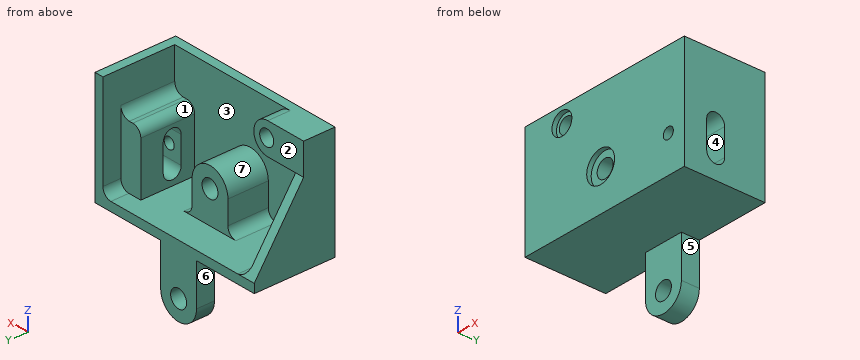
from build123d import *

# Parameters (mm, degrees)
BOSS_EXTRUDE1_DEPTH                                  = 6.35
BOSS_EXTRUDE2_DEPTH                                  = 57.15
BOSS_EXTRUDE3_DEPTH                                  = 44.45
BOSS_EXTRUDE4_DEPTH                                  = 34.925
SKETCH4_R                                            = 14.2875
SKETCH4_R_2                                          = 6.35
BOSS_EXTRUDE5_DEPTH                                  = 12.7
CUT_EXTRUDE1_REACH                                   = 159.28
BOSS_EXTRUDE6_DEPTH                                  = 15.875
CBORE_FOR_M5_CROSS_RECESS_PAN_HEAD_SCREW_D           = 11.2014
CBORE_FOR_M5_CROSS_RECESS_PAN_HEAD_SCREW_CBORE_D     = 15.875
CBORE_FOR_M5_CROSS_RECESS_PAN_HEAD_SCREW_CBORE_DEPTH = 3.175
CBORE_FOR_M5_CROSS_RECESS_PAN_HEAD_S_2_D             = 12.7
CBORE_FOR_M5_CROSS_RECESS_PAN_HEAD_S_2_CBORE_D       = 22.225
CBORE_FOR_M5_CROSS_RECESS_PAN_HEAD_S_2_CBORE_DEPTH   = 3.175
CUT_EXTRUDE3_REACH                                   = 159.28
CUT_EXTRUDE4_REACH                                   = 116.252
SKETCH18_R                                           = 4.0005


with BuildPart() as part:
    # Sketch1 → Boss-Extrude1 (new body)
    with BuildSketch(Plane(origin=(0, 0, 0), x_dir=(1, 0, 0), z_dir=(0, 1, 0))):
        with BuildLine():
            Line((60.325, 16.51822322), (60.325, -28.346886894))
            Line((60.325, -28.346886894), (60.325, -50.8))
            Line((60.325, -50.8), (66.675, -50.8))
            Line((66.675, -50.8), (66.675, 29.21822322))
            Line((66.675, 29.21822322), (-60.325, 29.21822322))
            Line((-60.325, 29.21822322), (-60.325, -50.8))
            Line((-60.325, -50.8), (-53.975, -50.8))
            Line((-53.975, -50.8), (-53.975, -44.45))
            Line((-53.975, -44.45), (-53.975, 16.103113106))
            ThreePointArc((-53.975, 16.103113106), (-51.993545123, 20.886768343), (-47.209889886, 22.86822322))
            Line((-47.209889886, 22.86822322), (-20.6375, 22.86822322))
            Line((-20.6375, 22.86822322), (20.6375, 22.86822322))
            Line((20.6375, 22.86822322), (44.45, 22.86822322))
            Line((44.45, 22.86822322), (53.975, 22.86822322))
            ThreePointArc((53.975, 22.86822322), (58.465128061, 21.00835128), (60.325, 16.51822322))
        make_face()
        with BuildLine():
            Line((60.325, -50.8), (60.325, -28.346886894))
            ThreePointArc((60.325, -28.346886894), (58.343545123, -23.563231657), (53.559889886, -21.58177678))
            Line((53.559889886, -21.58177678), (50.8, -21.58177678))
            ThreePointArc((50.8, -21.58177678), (46.309871939, -19.721904841), (44.45, -15.23177678))
            Line((44.45, -15.23177678), (44.45, 22.86822322))
            Line((44.45, 22.86822322), (20.6375, 22.86822322))
            ThreePointArc((20.6375, 22.86822322), (16.147371939, 21.00835128), (14.2875, 16.51822322))
            Line((14.2875, 16.51822322), (14.2875, 0))
            ThreePointArc((14.2875, 0), (0, -14.2875), (-14.2875, 0))
            Line((-14.2875, 0), (-14.2875, 16.51822322))
            ThreePointArc((-14.2875, 16.51822322), (-16.147371939, 21.00835128), (-20.6375, 22.86822322))
            Line((-20.6375, 22.86822322), (-47.209889886, 22.86822322))
            ThreePointArc((-47.209889886, 22.86822322), (-51.993545123, 20.886768343), (-53.975, 16.103113106))
            Line((-53.975, 16.103113106), (-53.975, -44.45))
            Line((-53.975, -44.45), (-53.975, -50.8))
            Line((-53.975, -50.8), (-47.625, -50.8))
            Line((-47.625, -50.8), (60.325, -50.8))
        make_face()
        with BuildLine():
            Line((-20.6375, 22.86822322), (20.6375, 22.86822322))
            ThreePointArc((20.6375, 22.86822322), (16.147371939, 21.00835128), (14.2875, 16.51822322))
            Line((14.2875, 16.51822322), (14.2875, 0))
            ThreePointArc((14.2875, 0), (0, -14.2875), (-14.2875, 0))
            Line((-14.2875, 0), (-14.2875, 16.51822322))
            ThreePointArc((-14.2875, 16.51822322), (-16.147371939, 21.00835128), (-20.6375, 22.86822322))
        make_face()
        with BuildLine():
            ThreePointArc((53.559889886, -21.58177678), (58.343545123, -23.563231657), (60.325, -28.346886894))
            Line((60.325, -28.346886894), (60.325, 16.51822322))
            ThreePointArc((60.325, 16.51822322), (58.465128061, 21.00835128), (53.975, 22.86822322))
            Line((53.975, 22.86822322), (44.45, 22.86822322))
            Line((44.45, 22.86822322), (44.45, -15.23177678))
            ThreePointArc((44.45, -15.23177678), (46.309871939, -19.721904841), (50.8, -21.58177678))
            Line((50.8, -21.58177678), (53.559889886, -21.58177678))
        make_face()
    extrude(amount=BOSS_EXTRUDE1_DEPTH)

    # Sketch1<4> → Boss-Extrude2 (add)
    with BuildSketch(Plane(origin=(0, 0, 0), x_dir=(1, 0, 0), z_dir=(0, 1, 0))):
        with BuildLine():
            Line((60.325, 16.51822322), (60.325, -28.346886894))
            Line((60.325, -28.346886894), (60.325, -50.8))
            Line((60.325, -50.8), (66.675, -50.8))
            Line((66.675, -50.8), (66.675, 29.21822322))
            Line((66.675, 29.21822322), (-60.325, 29.21822322))
            Line((-60.325, 29.21822322), (-60.325, -50.8))
            Line((-60.325, -50.8), (-53.975, -50.8))
            Line((-53.975, -50.8), (-53.975, -44.45))
            Line((-53.975, -44.45), (-53.975, 16.103113106))
            ThreePointArc((-53.975, 16.103113106), (-51.993545123, 20.886768343), (-47.209889886, 22.86822322))
            Line((-47.209889886, 22.86822322), (-20.6375, 22.86822322))
            Line((-20.6375, 22.86822322), (20.6375, 22.86822322))
            Line((20.6375, 22.86822322), (44.45, 22.86822322))
            Line((44.45, 22.86822322), (53.975, 22.86822322))
            ThreePointArc((53.975, 22.86822322), (58.465128061, 21.00835128), (60.325, 16.51822322))
        make_face()
    extrude(amount=BOSS_EXTRUDE2_DEPTH)

    # Sketch1<5> → Boss-Extrude3 (add)
    with BuildSketch(Plane(origin=(0, 0, 0), x_dir=(1, 0, 0), z_dir=(0, 1, 0))):
        with BuildLine():
            ThreePointArc((53.559889886, -21.58177678), (58.343545123, -23.563231657), (60.325, -28.346886894))
            Line((60.325, -28.346886894), (60.325, 16.51822322))
            ThreePointArc((60.325, 16.51822322), (58.465128061, 21.00835128), (53.975, 22.86822322))
            Line((53.975, 22.86822322), (44.45, 22.86822322))
            Line((44.45, 22.86822322), (44.45, -15.23177678))
            ThreePointArc((44.45, -15.23177678), (46.309871939, -19.721904841), (50.8, -21.58177678))
            Line((50.8, -21.58177678), (53.559889886, -21.58177678))
        make_face()
    extrude(amount=BOSS_EXTRUDE3_DEPTH)

    # Sketch1<6> → Boss-Extrude4 (add)
    with BuildSketch(Plane(origin=(0, 0, 0), x_dir=(1, 0, 0), z_dir=(0, 1, 0))):
        with BuildLine():
            Line((-20.6375, 22.86822322), (20.6375, 22.86822322))
            ThreePointArc((20.6375, 22.86822322), (16.147371939, 21.00835128), (14.2875, 16.51822322))
            Line((14.2875, 16.51822322), (14.2875, 0))
            ThreePointArc((14.2875, 0), (0, -14.2875), (-14.2875, 0))
            Line((-14.2875, 0), (-14.2875, 16.51822322))
            ThreePointArc((-14.2875, 16.51822322), (-16.147371939, 21.00835128), (-20.6375, 22.86822322))
        make_face()
    extrude(amount=BOSS_EXTRUDE4_DEPTH)

    # Sketch4 → Boss-Extrude5 (add)
    # profile 1 of 2: a face of its own
    with BuildSketch(Plane(origin=(0, 57.15, 0), x_dir=(1, 0, 0), z_dir=(0, 1, 0))):
        with BuildLine():
            ThreePointArc((14.2875, 58.801), (0, 44.5135), (-14.2875, 58.801))
            Line((-14.2875, 58.801), (-14.2875, 29.21822322))
            Line((-14.2875, 29.21822322), (14.2875, 29.21822322))
            Line((14.2875, 29.21822322), (14.2875, 58.801))
        make_face()
    # profile 2 of 2: a face of its own
    with BuildSketch(Plane(origin=(0, 57.15, 0), x_dir=(1, 0, 0), z_dir=(0, 1, 0))):
        with Locations((0, 58.801)):
            Circle(SKETCH4_R)
        with Locations(Location((0, 58.801, 0), (0, 0, 270))):
            Circle(SKETCH4_R_2, mode=Mode.SUBTRACT)
    extrude(amount=-BOSS_EXTRUDE5_DEPTH)

    # Sketch5 → Cut-Extrude1 (cut, up to next)
    with BuildSketch(Plane.ZY.offset(60.325), mode=Mode.PRIVATE) as cut_extrude1_sk1:
        Polygon((-22.86822322, 57.15), (28.575, 22.225), (50.8, 22.225), (50.8, 57.15), align=None)
    cut_extrude1_tool1 = extrude(cut_extrude1_sk1.sketch, amount=-CUT_EXTRUDE1_REACH, mode=Mode.PRIVATE) & part.part
    add(cut_extrude1_tool1.solids().sort_by_distance((-60.325, 42.810165, 24.526909))[0], mode=Mode.SUBTRACT)

    # Sketch6 → Boss-Extrude6 (add)
    with BuildSketch(Plane(origin=(0, 6.35, 0), x_dir=(1, 0, 0), z_dir=(0, 1, 0))):
        with BuildLine():
            Line((-31.75, -28.575), (-53.975, -28.575))
            Line((-53.975, -28.575), (-53.975, -50.8))
            Line((-53.975, -50.8), (-31.75, -50.8))
            ThreePointArc((-31.75, -50.8), (-20.6375, -39.6875), (-31.75, -28.575))
        make_face()
    extrude(amount=BOSS_EXTRUDE6_DEPTH)

    # CBORE for M5 Cross Recess Pan Head Screw (through all)
    with Locations(Plane(origin=(0, 0, 0), x_dir=(-1, 0, 0), z_dir=(0, -1, 0))):
        with Locations((30.873227599, -39.973489035)):
            CounterBoreHole(CBORE_FOR_M5_CROSS_RECESS_PAN_HEAD_SCREW_D / 2, CBORE_FOR_M5_CROSS_RECESS_PAN_HEAD_SCREW_CBORE_D / 2, CBORE_FOR_M5_CROSS_RECESS_PAN_HEAD_SCREW_CBORE_DEPTH)

    # CBORE for M5 Cross Recess Pan Head S 2 (through all)
    with Locations(Plane(origin=(0, 0, 0), x_dir=(-1, 0, 0), z_dir=(0, -1, 0))):
        with Locations((0, 0)):
            CounterBoreHole(CBORE_FOR_M5_CROSS_RECESS_PAN_HEAD_S_2_D / 2, CBORE_FOR_M5_CROSS_RECESS_PAN_HEAD_S_2_CBORE_D / 2, CBORE_FOR_M5_CROSS_RECESS_PAN_HEAD_S_2_CBORE_DEPTH)

    # Sketch16 → Cut-Extrude3 (cut, up to next)
    with BuildSketch(Plane(origin=(66.675, 0, 0), x_dir=(0, 0, -1), z_dir=(1, 0, 0)), mode=Mode.PRIVATE) as cut_extrude3_sk1:
        with BuildLine():
            Line((-6.35, 28.575), (12.7, 28.575))
            ThreePointArc((12.7, 28.575), (19.05, 22.225), (12.7, 15.875))
            Line((12.7, 15.875), (-6.35, 15.875))
            ThreePointArc((-6.35, 15.875), (-12.7, 22.225), (-6.35, 28.575))
        make_face()
    cut_extrude3_tool1 = extrude(cut_extrude3_sk1.sketch, amount=-CUT_EXTRUDE3_REACH, mode=Mode.PRIVATE) & part.part
    add(cut_extrude3_tool1.solids().sort_by_distance((66.675, 22.225, -3.175))[0], mode=Mode.SUBTRACT)

    # Sketch18 → Cut-Extrude4 (cut, up to next)
    with BuildSketch(Plane(origin=(0, 0, 0), x_dir=(-1, 0, 0), z_dir=(0, -1, 0)), mode=Mode.PRIVATE) as cut_extrude4_sk1:
        with Locations(Location((-53.975, 3.175, 0), (0, 0, 90))):
            Circle(SKETCH18_R)
    cut_extrude4_tool1 = extrude(cut_extrude4_sk1.sketch, amount=-CUT_EXTRUDE4_REACH, mode=Mode.PRIVATE) & part.part
    add(cut_extrude4_tool1.solids().sort_by_distance((53.975, 0, -3.175))[0], mode=Mode.SUBTRACT)


solid = part.part
Input: part model. Units: mm. Frame: model coordinates. Face numbers are marked on the shaded views. A direction names the side the tool comes from. Round coordinates to 2 decimals unless told otherwise and drop trailing zeros. Order: outer loops, then holes, each group sorted by start corner. A loop starts at its lowest first (then second) coordinate and runs counter-clockwise, first axis right, second up. Notation, with made-up numbers: (54, -26.75) - (113, -26.75) arc R22 cw to (113, -0.75) - close; hole circle Ø11 at (2.25, 61.5). An arc over 180 degrees is marked (long way). Answer as a JSON object with one key per item and string values. Group by question number.
(1) Draft query along Z for the marked faces 1, 2 and 3. Return one class per face: released by +Z, released by -Z, zero draft, split by the parting line, or undercut.
(2) Reachability of the marked faces 4, 5, 6 and 7 from +Z, -Z, +X, -X, +Y, -Y: full face, straight path, thin tool, end or side. Return the list, or none.
(3) Cut plane A-A (x = 0). Count the separate pieces of the cut face and the enclosed holes in it, then the cut area to 3 significant figures.
(4) Cut plane D-D (y = 42.5). Return loops of the section in (x, z) (3 decimals), then the cut area to 3 significant figures.
(5) Pin query (flat end, axial travel): P1, Ø5.5, axis at x = 55, z = -1.5, coming from the +Y side; P2, Ø0.8, axis at x = 53, y = 32.5, coming from the +Z side; P3, Ø23, axis at x = -3, z = -43.5, coming from the -Y side; P4, Ø13.5, axis at y = 25, z = 10, coming from the +X side (3 decimals). Return the tip coordinate at first contact, or that it passes through.
(6) Material intervals for probe 1 along Z at (x, y) = (0, 18.5); probe 2 along X at (y, z) = (19.5, 5) (3 decimals); probe 3 along X at (y, z) = (39, -6.5) (3 decimals), sorted ascending. Write a range as from..to.
(7) Cut plane C-C (x = 27). Return loops of the section in (y, z).
Here are the results:
{
 "1": {"face 1": "released by +Z", "face 2": "zero draft", "face 3": "undercut"},
 "2": {"face 4": "+X", "face 5": "-Z, +X, +Y, -Y", "face 6": "-Z, -X, +Y, -Y", "face 7": "+Z, +Y"},
 "3": {"separate pieces": "3", "enclosed holes": "0", "area": "1,810 mm^2"},
 "4": {"outline": "(-60.325, -29.218) - (66.675, -29.218) - (66.675, 50.8) - (60.325, 50.8) - (60.325, 28.347) arc R6.765 cw to (53.56, 21.582) - (50.8, 21.582) arc R6.35 ccw to (44.45, 15.232) - (44.45, -22.868) - (-47.21, -22.868) arc R6.765 cw to (-53.975, -16.103) - (-53.975, -1.289) - (-60.325, -1.289) - close", "area": "2,130 mm^2"},
 "5": {"P1": "stops at y = 44.45", "P2": "stops at z = 21.58", "P3": "stops at y = 44.45", "P4": "stops at x = 66.675"},
 "6": {"probe 1": "z = -29.22..-6.35, 6.35..14.29", "probe 2": "x = -60.325..-53.975, -13.384..-3.914, 3.914..13.384", "probe 3": "x = -60.325..-53.975, 44.45..66.675"},
 "7": {"outline": "(0, -29.22) - (57.15, -29.22) - (57.15, -22.87) - (6.35, -22.87) - (6.35, 50.8) - (0, 50.8) - close"}
}
